Part model, mm, in its own coordinate system. A direction names the side the tool comes from. Coordinates: 2 decimals unless noted, no trailing zeros. Order: outer loops, then holes, each group sorted by start corner. A loop starts at its lowest first (then second) coordinate and runs counter-clockwise, first axis right, second up.
1) Pin check, flat tips, straight feed: pin 1 Ø6 at (x, z) = (-36, -27) entering from +Y; pin 2 Ø2 at (y, z) = (-9.5, -45.5) entering from +X; pin 3 Ø8 at (x, z) = (-2, -146) entering from -Y. Stop position of each tip, or through.
2) Cut at A-A (z = 0). List the corners of the cut face in (x, y), and give its area (3 significant figures).
3) Tool access for faces 1 (the flat face through (50.095, 0.28, -171.005)), 2 (the flat face through (-145, 0, 0)), 3 (the cylindrical face through (-74.96, 0.28, -158.56)), 4 (the cylindrical face through (44.15, 34.3, -172.09)), 5 (the cylindrical face through (44.15, -34.3, -172.09)): list every direction of +Z, -Z, +X, -X, +Y, -Y with a clear straight run to the whole face (end or side of a thin tool).
4) Wall check: L1, parallel to Z at x = -57, y = -6; L2, parallel to Z at x = -41, y = -16; L3, parallel to Y at x = 32, z = -181. Give the ranges that are in metal, low to high.
```python
from build123d import *

# Parameters (mm, degrees)
F0_R          = 32.5
F1_DEPTH      = 85
F1_DEPTH_BACK = 145
F5_DEPTH      = 150
F7_W          = 125
F7_H          = 80
F8_DEPTH      = 50
F11_R         = 20
F12_R         = 4.99999


# Not quite as in the source:
# - a fillet or chamfer is up to 0.001 mm smaller than in the source, because OpenCascade refuses the exact size


with BuildPart() as f1:
    # F0 (on Right) → F1 (new body, two sides)
    with BuildSketch(Plane.YZ) as f1_sk:
        Circle(F0_R)
    extrude(amount=F1_DEPTH)
    extrude(f1_sk.sketch, amount=-F1_DEPTH_BACK)

    # F4 (on line) → F5 (join)
    with BuildSketch(Plane(origin=(0, 0, 0), x_dir=(0.9961946981, 0, 0.0871557427), z_dir=(0.0871557427, 0, -0.9961946981))):
        with BuildLine():
            add(Edge.make_bspline(
                [(25, 0), (25, 30.3108891325), (-12.5, 15.1554445662), (-50, 0), (-12.5, -15.1554445662), (25, -30.3108891325), (25, 0)],
                knots=[0, 0, 0, 2.0943951024, 2.0943951024, 4.1887902048, 4.1887902048, 6.2831853072, 6.2831853072, 6.2831853072], degree=2, weights=[1, 0.5, 1, 0.5, 1, 0.5, 1]))
        make_face()
    extrude(amount=F5_DEPTH)

    # F7 (on offset) → F8 (join)
    with BuildSketch(Plane(origin=(13.0733614121, 0, -149.4292047138), x_dir=(0.9961946981, 0, 0.0871557427), z_dir=(0.0871557427, 0, -0.9961946981))):
        with Locations((-27.5, 0)):
            Rectangle(F7_W, F7_H)
    extrude(amount=F8_DEPTH)

    # F9 (on Front) → F10 (revolve, cut)
    with BuildSketch(Plane.XZ):
        Polygon((-145, 32.5), (-145, 15.4653014615), (-99.2988270521, 32.5), align=None)
    revolve(axis=Axis((-67.4336478114, 0, 0), (1, 0, 0)), mode=Mode.SUBTRACT)

    # F11
    f11_edges = [f1.edges().sort_by_distance(p)[0] for p in [
        (-74.405268, 40, -182.178089),
        (-74.405268, -40, -182.178089),
        (50.119069, -40, -171.283621),
        (50.119069, 40, -171.283621),
    ]]
    fillet(f11_edges, radius=F11_R)

    # F12 (radius 5 in the source; OpenCascade refuses exactly that, so slightly less here)
    f12_edges = [f1.edges().sort_by_distance(p)[0] for p in [
        (-11.831506, 0, -151.608098),
        (47.940176, 0, -146.378754),
        (42.104602, 34.142136, -146.8893),
        (42.104602, -34.142136, -146.8893),
        (-14.321993, 40, -151.825988),
        (-14.321993, -40, -151.825988),
        (-70.748588, 34.142136, -156.762675),
        (-70.748588, -34.142136, -156.762675),
        (-76.584161, 0, -157.273222),
        (52.297963, 0, -196.188489),
        (46.46239, 34.142136, -196.699035),
        (46.46239, -34.142136, -196.699035),
        (-9.964206, 40, -201.635723),
        (-9.964206, -40, -201.635723),
        (-66.390801, 34.142136, -206.57241),
        (-66.390801, -34.142136, -206.57241),
        (-72.226374, 0, -207.082956),
    ]]
    fillet(f12_edges, radius=F12_R)


solid = f1.part
```
Geometry check:
1. pin 1: stops at y = 21.91
1. pin 2: stops at x = 25.92
1. pin 3: stops at y = -17.03
2. outline: (-145, -15.47) - (-99.3, -32.5) - (85, -32.5) - (85, 32.5) - (-99.3, 32.5) - (-145, 15.47) - close
2. area: 14,200 mm2
3. face 1: +X, +Y, -Y
3. face 2: +Z, -Z, -X, +Y, -Y
3. face 3: -X, +Y, -Y
3. face 4: +X, +Y
3. face 5: +X, -Y
4. L1: z = -205.75 to -155.56, -31.94 to 31.94
4. L2: z = -204.35 to -154.16, -28.29 to 28.29
4. L3: y = -39.97 to 39.97
